Study the drawing (mm; zero at the part's minimum x, y, z) and answer. A direction names the side the tool comes from. Round coordinates to 2 decimals unless told otherwise and drop trailing zeros. Write each loop counter-clockwise with the first axis right and the second up, starting at its lowest first coordinate (ties: lowest second). Pieces come first, ordered by that corner, then holes. Notation, with made-up numbers: M 51,38.25 L 95,38.25 A33 ccw 95,77.25 Z; hole C -8,23.25 d8. An arc over 180 degrees is marked long. Put each result on its own line as item: value. Start each with the question number.
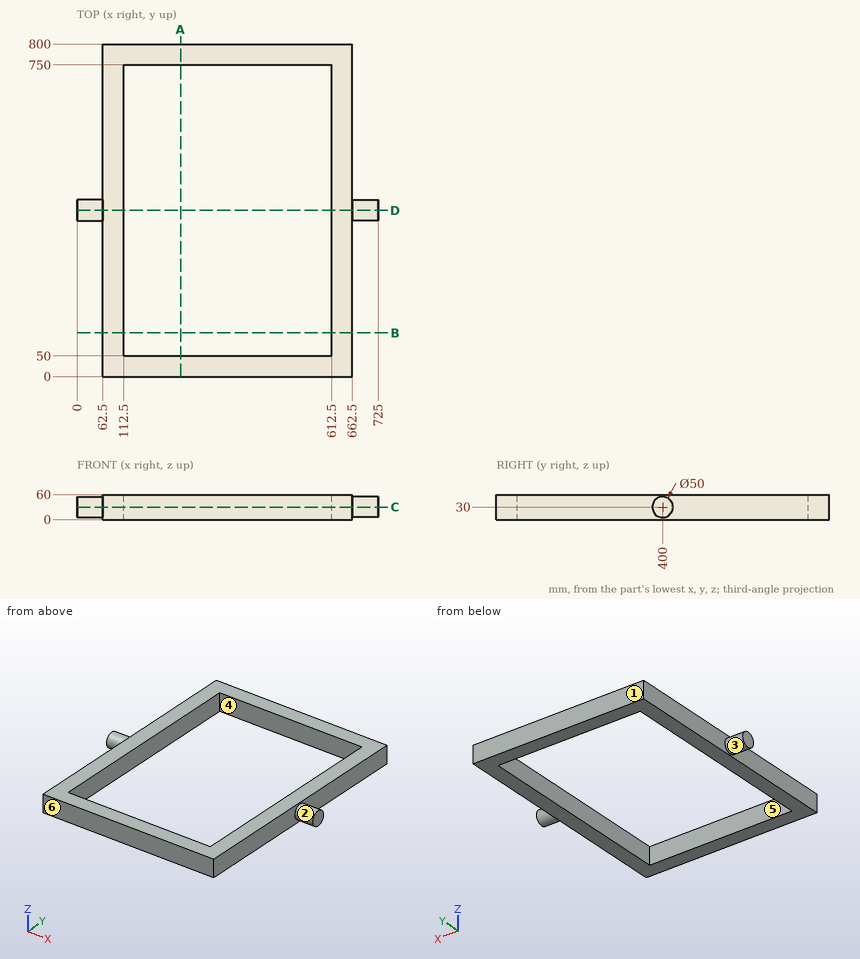
Item 1: Determine the mould class of the marked faces 3, 4, 5 and 6 for opening direction Y: released by +Y, released by -Y, zero draft, split by the parting line, or undercut.
Item 2: Section C-C (z = 30) is taken. Give the vertices of the cut face in (x, y), and give its area (3 significant figures).
Item 3: Which of the six approach directions +Z, -Z, +X, -X, +Y, -Y give full straight-line access (tool end or side, diameter ignored) to the marked faces 1 and 2?
Item 4: Consider line 1 along Y through (x, z) = (366.5, 8); line 2 along X through (y, z) = (555, 5.5); line 3 along X through (y, z) = (386.5, 26). Determine where each line is inside the solid, lowest interval first. Write a range as [from, to].
Item 5: Flat-ended cylindrical pins translate along their axes: pin 1 (1 mm diameter, centred on y = 540, z = 25, fed in from +X); pin 2 (2 mm diameter, centred on y = 184, z = 7, fed in from -X). Find the tip coordinate at first contact, or state that the pin passes through.
Item 6: Section D-D (y = 400) is taken. Give the vertices of the cut face in (x, z).
Item 7: Section B-B (y = 105) is taken. Give the vertices of the cut face in (x, z), and give its area (3 significant figures).
Item 8: Section A-A (x = 249) is taken. Give the vertices of the cut face in (y, z).
Output values:
1. face 3: split by the parting line
1. face 4: undercut
1. face 5: undercut
1. face 6: released by -Y
2. outline: M 0,375 L 62.5,375 L 62.5,0 L 662.5,0 L 662.5,375 L 725,375 L 725,425 L 662.5,425 L 662.5,800 L 62.5,800 L 62.5,425 L 0,425 Z; hole M 112.5,50 L 612.5,50 L 612.5,750 L 112.5,750 Z
2. area: 136,000 mm^2
3. face 1: +Z, -Z, +X, -X, +Y
3. face 2: +X
4. line 1: y = [0, 50], [750, 800]
4. line 2: x = [62.5, 112.5], [612.5, 662.5]
4. line 3: x = [0, 112.5], [612.5, 725]
5. pin 1: stops at x = 662.5
5. pin 2: stops at x = 62.5
6. outline: M 0,5 L 62.5,5 L 62.5,0 L 112.5,0 L 112.5,60 L 62.5,60 L 62.5,55 L 0,55 Z; M 612.5,0 L 662.5,0 L 662.5,5 L 725,5 L 725,55 L 662.5,55 L 662.5,60 L 612.5,60 Z
7. outline: M 62.5,0 L 112.5,0 L 112.5,60 L 62.5,60 Z; M 612.5,0 L 662.5,0 L 662.5,60 L 612.5,60 Z
7. area: 6,000 mm^2
8. outline: M 0,0 L 50,0 L 50,60 L 0,60 Z; M 750,0 L 800,0 L 800,60 L 750,60 Z
